from build123d import *

# Parameters (mm, degrees)
RESSALTO_EXTRUS_O4_DEPTH = 50
ESBO_O2_3_R              = 12
RESSALTO_EXTRUS_O5_DEPTH = 150


with BuildPart() as part:
    # Esbo_o2 → Ressalto-extrus_o4 (new body)
    with BuildSketch(Plane.XY):
        with BuildLine():
            Line((4, -14.313708499), (4, -11.313708499))
            ThreePointArc((4, -11.313708499), (0, -12), (-4, -11.313708499))
            Line((-4, -11.313708499), (-4, -14.313708499))
            Line((-4, -14.313708499), (4, -14.313708499))
        make_face()
    extrude(amount=RESSALTO_EXTRUS_O4_DEPTH)

    # Esbo_o2_3 → Ressalto-extrus_o5 (add)
    with BuildSketch(Plane.XY):
        Circle(ESBO_O2_3_R)
    extrude(amount=RESSALTO_EXTRUS_O5_DEPTH)


solid = part.part
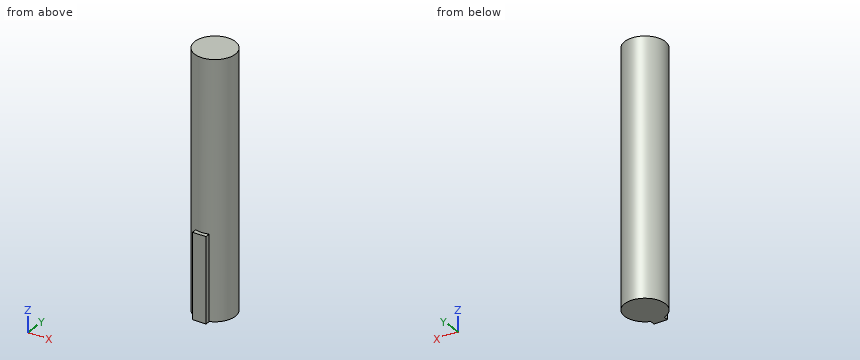
Geometry check sheet. Reference: the model listing, model coordinates, mm. Round coordinates to 2 decimals unless told otherwise and drop trailing zeros. Write each loop counter-clockwise with the first axis right and the second up, starting at its lowest first coordinate (ties: lowest second). Pieces come first, ordered by that corner, then holes. Notation, with made-up numbers: (-6.5, 65.5) -> (7.5, 65.5) arc R16 ccw to (7.5, 73.5) -> close; hole circle Ø3 at (55, 64). An arc over 180 degrees is marked (long way). One line per item, written item: value. Start each with the question number.
(1) Cross-section at D-D, the plane y = 5.25. Record the cut outline in (x, z).
(2) Go/stop test with flat-tipped pins: pin 1 Ø5 at (y, z) = (-3, 108) entering from -X; pin 2 Ø1.5 at (y, z) = (-12.5, 26) entering from -X; pin 3 Ø0.9 at (y, z) = (-13.5, 25) entering from +X. Record where each tip stops, or that it passes through.
(3) Scan lines: line 1 (X direction, y = 11, z = 93); line 2 (Y direction, x = -10, z = 61.5); line 3 (X direction, y = -1.75, z = 75.5). Record each from-to range of solid material in increasing order. Write a range as [from, to].
(4) Cross-section at C-C, the plane y = -9.5. Record the cut outline in (x, z).
(5) Cross-section at A-A, the plane x = 0. Record the cut outline in (y, z).
(6) Cross-section at B-B, the plane z = 99. Record the cut outline in (x, y).
Answer:
1. outline: (-10.79, 0) -> (10.79, 0) -> (10.79, 150) -> (-10.79, 150) -> close
2. pin 1: x = -11.99
2. pin 2: x = -4
2. pin 3: x = 4
3. line 1: [-4.8, 4.8]
3. line 2: [-6.63, 6.63]
3. line 3: [-11.87, 11.87]
4. outline: (-7.33, 0) -> (7.33, 0) -> (7.33, 150) -> (-7.33, 150) -> close
5. outline: (-14.31, 0) -> (12, 0) -> (12, 150) -> (-12, 150) -> (-12, 50) -> (-14.31, 50) -> close
6. outline: circle Ø24 at (0, 0)
